from build123d import *

# Parameters (mm, degrees)
F0_W     = 31.23
F0_H     = 28
F1_DEPTH = 13.3
F2_R     = 1.55
F3_DEPTH = 8.2


with BuildPart() as f1:
    # F0 (on Top) → F1 (new body)
    with BuildSketch(Plane.XY):
        Rectangle(F0_W, F0_H)
    extrude(amount=F1_DEPTH)

    # F2 (on face) → F3 (join)
    with BuildSketch(Plane.YZ.offset(15.615)):
        with Locations((0, 6.65)):
            Circle(F2_R)
    extrude(amount=F3_DEPTH)


solid = f1.part
Geometry check sheet. Reference: the model listing, model coordinates, mm. A direction names the side the tool comes from. Give positions to 0.01 mm unless a question says otherwise; leave off trailing zeros. Write each loop counter-clockwise with the first axis right and the second up, starting at its lowest first coordinate (ties: lowest second). Pieces come first, ordered by that corner, then holes.
1) Cross-section at A-A (y = 0). Record the boundary of the cut face in (x, z) (3 decimals).
Values follow:
outline: (-15.615, 0) - (15.615, 0) - (15.615, 5.1) - (23.815, 5.1) - (23.815, 8.2) - (15.615, 8.2) - (15.615, 13.3) - (-15.615, 13.3) - close
2) Thickness scan on line 1 (X direction, y = -7.5, z = 6.5) (3 decimals). Record the ranges inside material, lowest first.
Values follow:
line 1: x = -15.615 to 15.615
3) Cross-section at D-D (z = 2.25). Record the boundary of the cut face in (x, y) (3 decimals).
Values follow:
outline: (-15.615, -14) - (15.615, -14) - (15.615, 14) - (-15.615, 14) - close
4) Set-up check for faces 1 (the face through (19.658, -0.202, 8.187)), 2 (the face through (0, 0, 13.3)): record each of +Z, -Z, +X, -X, +Y, -Y from which the full face is reachable in a straight line by a thin tool's end or side.
Values follow:
face 1: +X
face 2: +Z, +X, -X, +Y, -Y
5) Cross-section at C-C (y = 6). Record the boundary of the cut face in (x, z) (3 decimals), plus the area to 3 significant figures.
Values follow:
outline: (-15.615, 0) - (15.615, 0) - (15.615, 13.3) - (-15.615, 13.3) - close
area: 415 mm2
6) Cross-section at B-B (z = 6.65). Record the boundary of the cut face in (x, y) (3 decimals).
Values follow:
outline: (-15.615, -14) - (15.615, -14) - (15.615, -1.55) - (23.815, -1.55) - (23.815, 1.55) - (15.615, 1.55) - (15.615, 14) - (-15.615, 14) - close
